Geometry: final body of the model. Coordinates: model frame, mm. A direction names the side the tool comes from. Round coordinates to 2 decimals unless told otherwise and drop trailing zeros. Loops run counter-clockwise (first coordinate to the right, second up) from the corner with the lowest first, then second, coordinate; pieces in that order, holes last. Notation, with made-up numbers: (-22, -24.5) - (32, -24.5) arc R14 ccw to (32, -6.5) - close; hole circle Ø6 at (45.25, 43). An arc over 180 degrees is marked (long way). Return JSON: item names as keys, results as strings. Group by question number.
1. Material intervals for probe 1 along Z at (x, y) = (0, 29); probe 2 along Y at (x, z) = (27, -49.5); probe 3 along X at (y, z) = (17.5, -2), sorted ascending.
2. Section C-C on y = 38.5. Return loops of the section in (x, z), and give its area (3 significant figures).
3. Section A-A on z = 0. Return loops of the section in (x, y).
4. Section D-D on x = -46. Return loops of the section in (y, z).
5. First-contact query: pin 1 Ø10 at (x, y) = (5, 26) entering from +Z; pin 2 Ø4 at (x, y) = (33.5, 29) entering from +Z; pin 3 Ø12 at (y, z) = (27, 37) entering from +X. Flat tips, straight axial feed; report the tip coordinate or a pass-through.
6. Section B-B on x = 0. Return loops of the section in (y, z).
7. Set-up query: faces 4 (the face through (-12, 40.612, 1)), 5 (the face through (-35.4, 10.612, -24.4)). Return all of +Z, -Z, +X, -X, +Y, -Y with unobstructed straight access to the full face (end or side cutting, diameter ignored); none if empty.
8. Draft query along Z for faces 1 (the face through (8, 35.612, 47)), 2 (the face through (-0.54, 25.09, -2.44)), 3 (the face through (12.465, 38.147, -56.133)). Return one class per face: +Z half, -Z half, draft (parallel to the pull), parting line (faces both ways), or undercut.
from build123d import *

# Parameters (mm, degrees)
SKETCH2_R          = 2.5
CUT_EXTRUDE1_DEPTH = 40


with BuildPart() as part:
    # Sketch1 → Revolve1 (revolve)
    with BuildSketch(Plane.XY):
        Polygon((0, 10), (-2.5, 10), (-12.682056098, 20.182056098), (-22.5, 10.364112197), (-32.623909355, 20.488021552), (-42.5, 10.611930908), (-47.5, 10.611930908), (-47.5, 35.611930908), (-57.5, 35.611930908), (-57.5, 40.611930908), (0, 40.611930908), align=None)
    revolve(axis=Axis((0, 40.611930908, 0), (0, 1, 0)))

    # Sketch2 → Cut-Extrude1 (cut)
    with BuildSketch(Plane.XZ.offset(-10)):
        Circle(SKETCH2_R)
    extrude(amount=-CUT_EXTRUDE1_DEPTH, mode=Mode.SUBTRACT)


solid = part.part
Taken from the geometry:
{
 "1": {"probe 1": "-47.5 to -2.5, 2.5 to 47.5", "probe 2": "35.61 to 40.61", "probe 3": "-47.46 to -35.56, -29.57 to -15.23, -9.8 to -1.5, 1.5 to 9.8, 15.23 to 29.57, 35.56 to 47.46"},
 "2": {"outline": "circle Ø115 at (0, 0); hole circle Ø5 at (0, 0)", "area": "10,400 mm2"},
 "3": {"outline": "(-57.5, 35.61) - (-47.5, 35.61) - (-47.5, 10.61) - (-42.5, 10.61) - (-32.62, 20.49) - (-22.5, 10.36) - (-12.68, 20.18) - (-2.5, 10) - (-2.5, 40.61) - (-57.5, 40.61) - close; (2.5, 10) - (12.68, 20.18) - (22.5, 10.36) - (32.62, 20.49) - (42.5, 10.61) - (47.5, 10.61) - (47.5, 35.61) - (57.5, 35.61) - (57.5, 40.61) - (2.5, 40.61) - close"},
 "4": {"outline": "(10.61, -11.84) - (35.61, -11.84) - (35.61, -34.5) - (40.61, -34.5) - (40.61, 34.5) - (35.61, 34.5) - (35.61, 11.84) - (10.61, 11.84) - close"},
 "5": {"pin 1": "z = 47.5", "pin 2": "z = 35.55", "pin 3": "x = 35.99"},
 "6": {"outline": "(10, -2.5) - (20.18, -12.68) - (10.36, -22.5) - (20.49, -32.62) - (10.61, -42.5) - (10.61, -47.5) - (35.61, -47.5) - (35.61, -57.5) - (40.61, -57.5) - (40.61, -2.5) - close; (10, 2.5) - (40.61, 2.5) - (40.61, 57.5) - (35.61, 57.5) - (35.61, 47.5) - (10.61, 47.5) - (10.61, 42.5) - (20.49, 32.62) - (10.36, 22.5) - (20.18, 12.68) - close"},
 "7": {"face 4": "+Z, -Z, +X, -X, +Y", "face 5": "-Y"},
 "8": {"face 1": "draft", "face 2": "undercut", "face 3": "parting line"}
}
